The listing builds one solid part. Answer for the finished solid, in the listing's coordinates (mm). Face numbers are marked on the shaded views. A direction names the side the tool comes from. Coordinates: 2 decimals unless noted, no trailing zeros. Order: outer loops, then holes, each group sorted by start corner. A loop starts at its lowest first (then second) coordinate and runs counter-clockwise, first axis right, second up. Notation, with made-up numbers: (56.25, 38.5) -> (74.25, 38.5) arc R25 cw to (74.25, 59.5) -> close; hole circle Ø7 at (-35.5, 80.25). An arc over 180 degrees is marked (long way). Return JSON: item names as keys, results as strings.
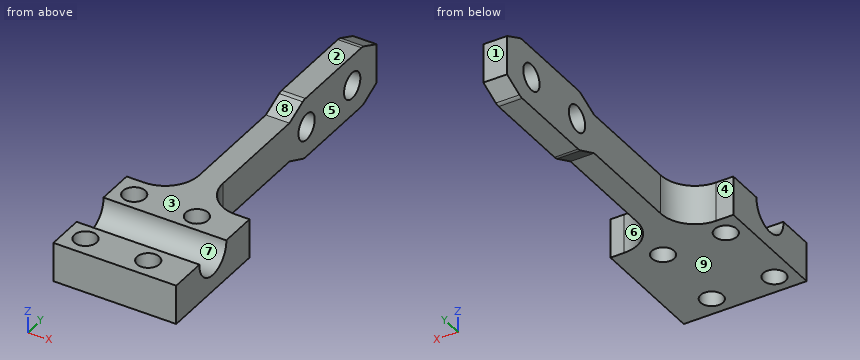
from build123d import *

# Parameters (mm, degrees)
SKETCH1_R           = 4.25
BOSS_EXTRUDE1_DEPTH = 15
SKETCH3_R           = 8.25
CUT_EXTRUDE1_DEPTH  = 55.05
SKETCH4_R           = 5
CUT_EXTRUDE3_DEPTH  = 46.05
BOSS_EXTRUDE2_DEPTH = 9
FILLET1_R           = 13


with BuildPart() as part:
    # Sketch1 → Boss-Extrude1 (new body)
    with BuildSketch(Plane.XY):
        with BuildLine():
            Line((-8.1, 22.5), (-8.1, 129.9))
            Line((-8.1, 129.9), (0.9, 129.9))
            Line((0.9, 129.9), (0.9, 35.5))
            ThreePointArc((0.9, 35.5), (4.707611845, 26.307611845), (13.9, 22.5))
            Line((13.9, 22.5), (20.5, 22.5))
            Line((20.5, 22.5), (20.5, -22.5))
            Line((20.5, -22.5), (-26.3, -22.5))
            Line((-26.3, -22.5), (-26.3, 22.5))
            Line((-26.3, 22.5), (-8.1, 22.5))
        make_face()
        with Locations((-10.95, -14.95)):
            Circle(SKETCH1_R, mode=Mode.SUBTRACT)
        with Locations((12.95, -14.95)):
            Circle(SKETCH1_R, mode=Mode.SUBTRACT)
        with Locations((12.95, 14.95)):
            Circle(SKETCH1_R, mode=Mode.SUBTRACT)
        with Locations((-10.95, 14.95)):
            Circle(SKETCH1_R, mode=Mode.SUBTRACT)
    extrude(amount=BOSS_EXTRUDE1_DEPTH)

    # Sketch3 → Cut-Extrude1 (cut)
    with BuildSketch(Plane.ZY.offset(26.3)):
        with Locations((14.5, 0)):
            Circle(SKETCH3_R)
    extrude(amount=-CUT_EXTRUDE1_DEPTH, mode=Mode.SUBTRACT)

    # Sketch4 → Cut-Extrude3 (cut)
    with BuildSketch(Plane(origin=(0.9, 0, 0), x_dir=(0, 0, -1), z_dir=(1, 0, 0))):
        with Locations((-7.5, 86.9)):
            Circle(SKETCH4_R)
        with Locations((-7.5, 114.9)):
            Circle(SKETCH4_R)
    extrude(amount=-CUT_EXTRUDE3_DEPTH, mode=Mode.SUBTRACT)

    # Sketch6 → Boss-Extrude2 (add)
    with BuildSketch(Plane.ZY.offset(8.1)):
        with BuildLine():
            Line((15, 76.386851455), (18.651630299, 84.554112306))
            ThreePointArc((18.651630299, 84.554112306), (18.911938215, 85.352068488), (19, 86.186777661))
            Line((19, 86.186777661), (19, 120.550049196))
            ThreePointArc((19, 120.550049196), (18.902685036, 121.427003874), (18.615475246, 122.261288146))
            Line((18.615475246, 122.261288146), (15, 129.9))
            Line((15, 129.9), (15, 76.386851455))
        make_face()
        with BuildLine():
            Line((-3.615475246, 122.261288146), (0, 129.9))
            Line((0, 129.9), (0, 76.386851455))
            Line((0, 76.386851455), (-3.651630299, 84.554112306))
            ThreePointArc((-3.651630299, 84.554112306), (-3.911938215, 85.352068488), (-4, 86.186777661))
            Line((-4, 86.186777661), (-4, 120.550049196))
            ThreePointArc((-4, 120.550049196), (-3.902685036, 121.427003874), (-3.615475246, 122.261288146))
        make_face()
    extrude(amount=-BOSS_EXTRUDE2_DEPTH)

    # Fillet1
    fillet1_edges = [part.edges().sort_by_distance(p)[0] for p in [
        (-8.1, 22.5, 7.5),
    ]]
    fillet(fillet1_edges, radius=FILLET1_R)


with BuildPart() as body_2:
    # Mirror2: mirrored copy
    add(part.part.mirror(Plane(origin=(20.5, -22.5, 15), x_dir=(0, 0, 1), z_dir=(-1, 0, 0))))


solid = body_2.part
1. Determine the mould class of the marked faces 6, 7, 8 and 9 for opening direction Y: pulls with the +Y half, pulls with the -Y half, needs draft (parallel to the pull), parting line crosses it, or undercut.
Answer block:
{"face 6": "pulls with the +Y half", "face 7": "undercut", "face 8": "pulls with the -Y half", "face 9": "needs draft"}
2. For the marked faces 1, 2, 3, 4 and 5, determine the directions among +Z, -Z, +X, -X, +Y, -Y from which every point of the face is accessible in a straight line to the end or side of a thin tool.
Answer block:
{"face 1": "+Z, -Z, +X, -X, +Y", "face 2": "+Z, +X, -X, +Y, -Y", "face 3": "+Z, +X, -X, -Y", "face 4": "+Z, -Z, -X, +Y", "face 5": "+Z, -Z, +X, +Y"}
3. The part is cut by section C-C on y = 114.9. Give the vertices of the cut face in (x, z).
Answer block:
{"outline": "(40.1, -4) -> (49.1, -4) -> (49.1, 2.5) -> (40.1, 2.5) -> close; (40.1, 12.5) -> (49.1, 12.5) -> (49.1, 19) -> (40.1, 19) -> close"}
4. Each of these flat-tipped pins is pushed along its axis until it touches: pin 1 Ø12 at (y, z) = (30, 2) entering from -X; pin 2 Ø4.5 at (x, y) = (33.5, -12.5) entering from +Z; pin 3 Ø3.5 at (x, z) = (23, 7.5) entering from +Y. Where does it stop, or does it pass through?
Answer block:
{"pin 1": "stops at x = 33.16", "pin 2": "stops at z = 15", "pin 3": "stops at y = 22.5"}
5. The part is cut by section A-A on y = -14.95. Give the vertices of the cut face in (x, z).
Answer block:
{"outline": "(20.5, 0) -> (23.8, 0) -> (23.8, 15) -> (20.5, 15) -> close; (32.3, 0) -> (47.7, 0) -> (47.7, 15) -> (32.3, 15) -> close; (56.2, 0) -> (67.3, 0) -> (67.3, 15) -> (56.2, 15) -> close"}
6. Consider line 1 (Z direction, x = 41, y = 114.5); line 2 (Y direction, x = 51.95, z = 11.25); line 3 (Y direction, x = 51.95, z = 4.75). Determine where each line is inside the solid, lowest interval first. Write a range as from..to.
Answer block:
{"line 1": "z = -4..2.52, 12.48..19", "line 2": "y = -22.5..-19.2, -10.7..-7.58, 7.58..10.7, 19.2..27.38", "line 3": "y = -22.5..-19.2, -10.7..10.7, 19.2..27.38"}
7. The part is cut by section B-B on z = 10. Give the vertices of the cut face in (x, y), and give its area (3 significant figures).
Answer block:
{"outline": "(20.5, -22.5) -> (67.3, -22.5) -> (67.3, -6.91) -> (20.5, -6.91) -> close; (20.5, 6.91) -> (67.3, 6.91) -> (67.3, 22.5) -> (62.1, 22.5) arc R13 cw to (49.1, 35.5) -> (49.1, 82.57) -> (40.1, 82.57) -> (40.1, 35.5) arc R13 cw to (27.1, 22.5) -> (20.5, 22.5) -> close; (40.1, 91.23) -> (49.1, 91.23) -> (49.1, 110.57) -> (40.1, 110.57) -> close; (40.1, 119.23) -> (49.1, 119.23) -> (49.1, 129.9) -> (40.1, 129.9) -> close; hole circle Ø8.5 at (28.05, -14.95); hole circle Ø8.5 at (28.05, 14.95); hole circle Ø8.5 at (51.95, -14.95); hole circle Ø8.5 at (51.95, 14.95)", "area": "2,120 mm2"}
8. The part is cut by section D-D on x = 35. Give the vertices of the cut face in (y, z).
Answer block:
{"outline": "(-22.5, 0) -> (25.18, 0) -> (25.18, 15) -> (8.23, 15) arc R8.25 cw (long way) to (-8.23, 15) -> (-22.5, 15) -> close"}
